Design review of the part built by this model. Coordinates are the model's own, in mm. A direction names the side the tool comes from. Round coordinates to 2 decimals unless told otherwise and drop trailing zeros. Order: outer loops, then holes, each group sorted by start corner. A loop starts at its lowest first (then second) coordinate and runs counter-clockwise, first axis right, second up. Notation, with made-up numbers: (-8.5, 67.25) - (2.5, 67.25) arc R15 ccw to (2.5, 79.25) - close; hole circle Ø6 at (-14, -16.5). An arc over 180 degrees is marked (long way). Write item = value, one per line.
from build123d import *

# Parameters (mm, degrees)
SKETCH1_R           = 4.2
BOSS_EXTRUDE1_DEPTH = 8
FILLET1_R           = 10
CHAMFER1_SIZE       = 0.5


with BuildPart() as part:
    # Sketch1 → Boss-Extrude1 (new body)
    with BuildSketch(Plane(origin=(0, 0, 0), x_dir=(1, 0, 0), z_dir=(0, 1, 0))):
        with BuildLine():
            Line((-4, 28.73484861), (-4, -28.73484861))
            ThreePointArc((-4, -28.73484861), (0, -47.9), (4, -28.73484861))
            Line((4, -28.73484861), (4, 28.73484861))
            ThreePointArc((4, 28.73484861), (0, 47.9), (-4, 28.73484861))
        make_face()
        with Locations((0, 37.9)):
            Circle(SKETCH1_R, mode=Mode.SUBTRACT)
        with Locations((0, -37.9)):
            Circle(SKETCH1_R, mode=Mode.SUBTRACT)
    extrude(amount=BOSS_EXTRUDE1_DEPTH)

    # Fillet1
    fillet1_edges = [part.edges().sort_by_distance(p)[0] for p in [
        (4, 4, -28.73484861),
        (4, 4, 28.73484861),
        (-4, 4, 28.73484861),
        (-4, 4, -28.73484861),
    ]]
    fillet(fillet1_edges, radius=FILLET1_R)

    # Chamfer1
    chamfer1_edges = [part.edges().sort_by_distance(p)[0] for p in [
        (-4.2, 0, -37.9),
        (-4.2, 8, -37.9),
        (-4.2, 0, 37.9),
        (-4.2, 8, 37.9),
        (4, 0, 0),
        (4, 8, 0),
        (0, 0, 47.9),
        (0, 8, 47.9),
        (0, 0, -47.9),
        (0, 8, -47.9),
        (-4, 0, 0),
        (-4, 8, 0),
        (4.780455543, 0, 27.490126489),
        (4.780455543, 8, 27.490126489),
        (4.780455543, 0, -27.490126489),
        (4.780455543, 8, -27.490126489),
        (-4.780455543, 0, -27.490126489),
        (-4.780455543, 8, -27.490126489),
        (-4.780455543, 0, 27.490126489),
        (-4.780455543, 8, 27.490126489),
    ]]
    chamfer(chamfer1_edges, length=CHAMFER1_SIZE)


solid = part.part
1) Clearance check with flat-ended pins moving along their axes: pin 1 Ø1.5 at (y, z) = (6, -23) entering from +X; pin 2 Ø6.5 at (x, z) = (0, 37.9) entering from -Y; pin 3 Ø2 at (y, z) = (5.5, -11.5) entering from -X; pin 4 Ø4 at (x, y) = (2.5, 1) entering from -Z. State where each tip first meets the part, or that it passes through.
Findings:
pin_1 = 4
pin_2 = through
pin_3 = -4
pin_4 = -47.89
2) We need section C-C on y = 4.75. Write out the cut boundary in (x, z), and give its area (3 significant figures).
Findings:
outline = (-7, -30.76) arc R10 ccw (long way) to (7, -30.76) arc R10 cw to (4, -23.62) - (4, 23.62) arc R10 cw to (7, 30.76) arc R10 ccw (long way) to (-7, 30.76) arc R10 cw to (-4, 23.62) - (-4, -23.62) arc R10 cw to start; hole circle Ø8.4 at (0, -37.9); hole circle Ø8.4 at (0, 37.9)
area = 981 mm^2
3) We need section B-B on z = -37.9. Write out the cut boundary in (x, y), and give its area (3 significant figures).
Findings:
outline = (-10, 0.5) - (-9.5, 0) - (-4.7, 0) - (-4.2, 0.5) - (-4.2, 7.5) - (-4.7, 8) - (-9.5, 8) - (-10, 7.5) - close; (4.2, 0.5) - (4.7, 0) - (9.5, 0) - (10, 0.5) - (10, 7.5) - (9.5, 8) - (4.7, 8) - (4.2, 7.5) - close
area = 91.8 mm^2
4) The part is to be moulded in two halves that separate along Z. For faces 3 (the cylindrical face through (2.26, 3.95, -41.44)), 4 (the flat face through (-4, 4, 0)), 5 (the flat face through (0, 8, -1)), say which applies: released by +Z, released by -Z, zero draft, split by the parting line, or undercut.
Findings:
face_3 = undercut
face_4 = undercut
face_5 = zero draft
5) We need section A-A on x = 0. Write out the cut boundary in (y, z).
Findings:
outline = (0, -47.4) - (0.5, -47.9) - (7.5, -47.9) - (8, -47.4) - (8, -42.6) - (7.5, -42.1) - (0.5, -42.1) - (0, -42.6) - close; (0, -33.2) - (0.5, -33.7) - (7.5, -33.7) - (8, -33.2) - (8, 33.2) - (7.5, 33.7) - (0.5, 33.7) - (0, 33.2) - close; (0, 42.6) - (0.5, 42.1) - (7.5, 42.1) - (8, 42.6) - (8, 47.4) - (7.5, 47.9) - (0.5, 47.9) - (0, 47.4) - close
6) For faces 1 (the flat face through (4, 4, 0)), 2 (the cylindrical face through (1.938, 3.951, 41.626)), list the 3-axis set-ups (+Z, -Z, +X, -X, +Y, -Y) from which the entire face can be reached by the end or side of a thin tool; tool diameter is ignored.
Findings:
face_1 = +X, +Y, -Y
face_2 = +Y, -Y
7) To check wall thickness, follow L1, parallel to X at y = 2, z = 37.9; L2, parallel to Z at x = -2, y = 2.25; L3, parallel to X at y = 6.5, z = -10.5. State the ranges of each line that lie inside material, in increasing order. Write a range as from..to.
Findings:
L1 = -10..-4.2, 4.2..10
L2 = -47.7..-41.59, -34.21..34.21, 41.59..47.7
L3 = -4..4
8) We need section D-D on z = -3. Write out the cut boundary in (x, y).
Findings:
outline = (-4, 0.5) - (-3.5, 0) - (3.5, 0) - (4, 0.5) - (4, 7.5) - (3.5, 8) - (-3.5, 8) - (-4, 7.5) - close
